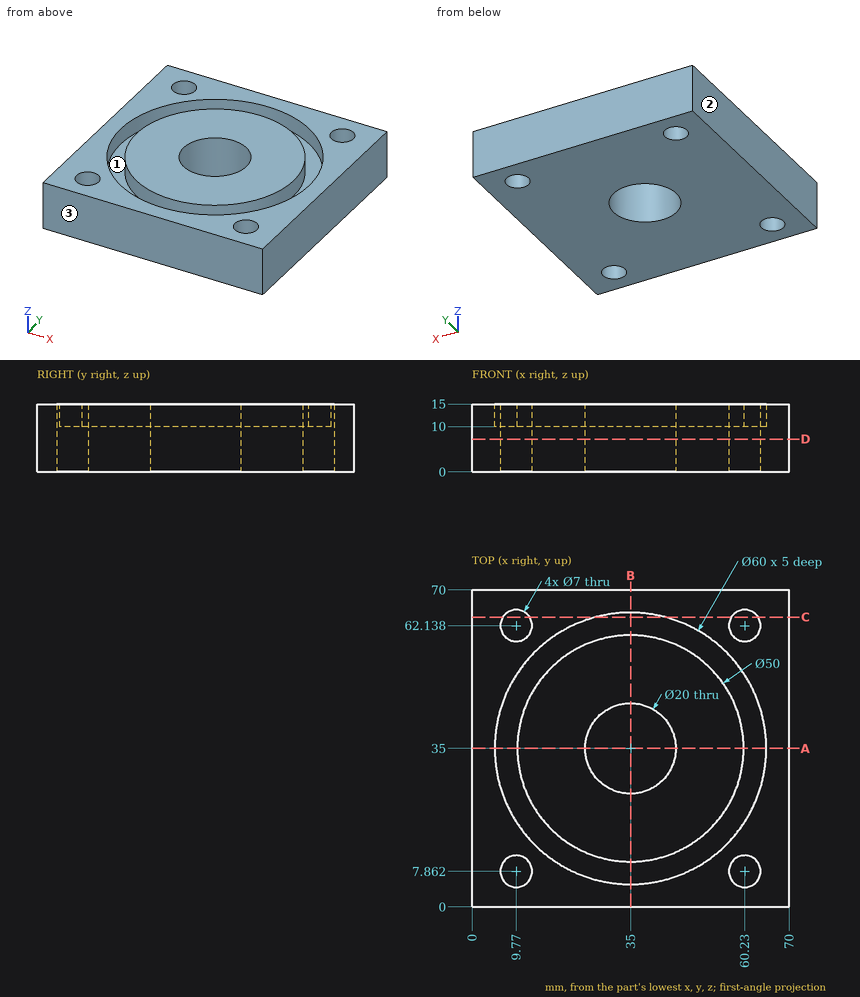
Verification items for this drawing (mm, ordinates from the low corner). Give positions to 0.01 mm unless a question says otherwise; leave off trailing zeros. Loops run counter-clockwise (first coordinate to the right, second up) from the corner with the lowest first, then second, coordinate; pieces in that order, holes last. Notation, with made-up numbers: M 46.25,80 L 86.25,80 A20 cw 86.25,115 Z; hole C 60,4.5 d7. An arc over 180 degrees is marked long. Answer as CSV lines item,"result".
Item 1: Cross-section at D-D on z = 7.25. Record the cut outline in (x, y), and give its area (3 significant figures).
Values:
outline,"M 0,0 L 70,0 L 70,70 L 0,70 Z; hole C 9.77,7.86 d7; hole C 9.77,62.14 d7; hole C 35,35 d20; hole C 60.23,7.86 d7; hole C 60.23,62.14 d7"
area,"4,430 mm²"
Item 2: Cross-section at A-A on y = 35. Record the cut outline in (x, z).
Values:
outline,"M 0,0 L 25,0 L 25,15 L 10,15 L 10,10 L 5,10 L 5,15 L 0,15 Z; M 45,0 L 70,0 L 70,15 L 65,15 L 65,10 L 60,10 L 60,15 L 45,15 Z"
Item 3: Cross-section at C-C on y = 64. Record the cut outline in (x, z).
Values:
outline,"M 0,0 L 6.81,0 L 6.81,15 L 0,15 Z; M 12.73,0 L 57.27,0 L 57.27,15 L 42.68,15 L 42.68,10 L 27.32,10 L 27.32,15 L 12.73,15 Z; M 63.19,0 L 70,0 L 70,15 L 63.19,15 Z"
Item 4: Material ranges on line 1 (X direction, y = 62.5, z = 2.75); line 2 (X direction, y = 10.5, z = 7); line 3 (Y direction, x = 38, z = 11.75), recorded low to high.
Values:
line 1,"x = 0 to 6.29, 13.25 to 56.75, 63.71 to 70"
line 2,"x = 0 to 7.47, 12.07 to 57.93, 62.53 to 70"
line 3,"y = 0 to 5.15, 10.18 to 25.46, 44.54 to 59.82, 64.85 to 70"
Item 5: Release check for a two-part mould opening along X. For the marked faces 1, 2 and 3 record: pulls with the +X half, pulls with the -X half, needs draft (parallel to the pull), parting line crosses it, or undercut.
Values:
face 1,"undercut"
face 2,"pulls with the -X half"
face 3,"needs draft"
